Build history of the part. All positions in model axes, mm. Give positions to 0.01 mm unless a question says otherwise; leave off trailing zeros. Loops run counter-clockwise (first coordinate to the right, second up) from the corner with the lowest first, then second, coordinate; pieces in that order, holes last. Notation, with made-up numbers: M 0,86 L 53,86 A18 cw 53,115 Z; hole C 22,-23 d1. An arc over 180 degrees is marked long. Answer as a JSON object with one key per item and string values. Group by question number.
1. Drill centre lines: line 1 along Y through (x, z) = (8, 6.5); line 2 along X through (y, z) = (-54, -9.75); line 3 along X through (y, z) = (51, -2). Where is each one in solid material? Low to high. Write a range as [from, to].
2. Slice it at A-A (x = -54.5). List the corners of the cut face in (y, z), then the cut area to 3 significant figures.
3. Slice it at B-B (y = -20). List the corners of the cut face in (x, z), then the cut area to 3 significant figures.
4. Mould opens along Y. For faces 1 (the face through (-6, 54.193, 0)), 2 (the face through (31, 7.468, 0)) say: released by +Y, released by -Y, zero draft, split by the parting line, or undercut.
5. Slice it at D-D (x = -26). List the corners of the cut face in (y, z), then the cut area to 3 significant figures.
6. Slice it at C-C (z = -4.25). Give the number of separate pieces and of enclosed holes in the cut face, then the cut area to 3 significant figures.
7. Drop flat-ended pins along their axis: pin 1 Ø2 at (x, z) = (-5, 5) entering from -Y; pin 2 Ø2 at (x, z) = (6, -1.5) entering from -Y; pin 3 Ø5 at (y, z) = (19.5, 6) entering from +X. Give the stop position or say it passes through.
from build123d import *

# Parameters (mm, degrees)
F0_W     = 34.350958
F0_H     = 4.69392
F0_W_2   = 4.2672
F0_H_2   = 36.697921
F0_W_3   = 32.217363
F0_W_4   = 4.480557
F0_H_3   = 37.12464
F0_H_4   = 34.350963
F0_H_5   = 4.05384
F1_DEPTH = 11.176


with BuildPart() as f1:
    # F0 (on Top) → F1 (new body, symmetric)
    with BuildSketch(Plane.XY):
        with BuildLine():
            ThreePointArc((-12.7, 0), (-8.980256, 8.980256), (0, 12.7))
            Line((0, 12.7), (0, 76.2))
            ThreePointArc((0, 76.2), (-53.881537, 53.881537), (-76.2, 0))
            Line((-76.2, 0), (-12.7, 0))
        make_face()
        with BuildLine():
            Line((-49.08218, 40.288828), (-17.906999, 12.7))
            Line((-17.906999, 12.7), (-62.217039, 12.7))
            ThreePointArc((-62.217039, 12.7), (-57.333802, 27.296247), (-49.08218, 40.288828))
        make_face(mode=Mode.SUBTRACT)
        with Locations((-33.588959, 5.12064)):
            Rectangle(F0_W, F0_H, mode=Mode.SUBTRACT)
        with Locations((-5.958838, 35.844481)):
            Rectangle(F0_W_2, F0_H_2, mode=Mode.SUBTRACT)
        with BuildLine():
            ThreePointArc((-44.31846, 45.476633), (-29.712564, 56.119636), (-12.7, 62.217039))
            Line((-12.7, 62.217039), (-12.7, 17.49552))
            Line((-12.7, 17.49552), (-44.31846, 45.476633))
        make_face(mode=Mode.SUBTRACT)
        with BuildLine():
            ThreePointArc((0, 12.7), (8.980256, 8.980256), (12.7, 0))
            Line((12.7, 0), (76.2, 0))
            ThreePointArc((76.2, 0), (53.881537, 53.881537), (0, 76.2))
            Line((0, 76.2), (0, 12.7))
        make_face()
        with Locations((31.485843, 5.12064)):
            Rectangle(F0_W_3, F0_H, mode=Mode.SUBTRACT)
        with Locations((6.096001, 35.631121)):
            Rectangle(F0_W_4, F0_H_3, mode=Mode.SUBTRACT)
        with BuildLine():
            Line((62.217039, 12.7), (17.724123, 12.7))
            Line((17.724123, 12.7), (42.179105, 47.467601))
            ThreePointArc((42.179105, 47.467601), (55.016682, 31.708276), (62.217039, 12.7))
        make_face(mode=Mode.SUBTRACT)
        with BuildLine():
            Line((36.695692, 51.82351), (12.7, 17.708881))
            Line((12.7, 17.708881), (12.7, 62.217039))
            ThreePointArc((12.7, 62.217039), (25.23866, 58.26886), (36.695692, 51.82351))
        make_face(mode=Mode.SUBTRACT)
        with BuildLine():
            Line((76.2, 0), (12.7, 0))
            ThreePointArc((12.7, 0), (8.980256, -8.980256), (0, -12.7))
            Line((0, -12.7), (0, -76.2))
            ThreePointArc((0, -76.2), (53.881537, -53.881537), (76.2, 0))
        make_face()
        with BuildLine():
            Line((12.7, -62.217039), (12.7, -17.068801))
            Line((12.7, -17.068801), (39.648922, -49.600534))
            ThreePointArc((39.648922, -49.600534), (26.923901, -57.509595), (12.7, -62.217039))
        make_face(mode=Mode.SUBTRACT)
        with Locations((6.096001, -33.390842)):
            Rectangle(F0_W_4, F0_H_4, mode=Mode.SUBTRACT)
        with Locations((31.485843, -4.58724)):
            Rectangle(F0_W_3, F0_H_5, mode=Mode.SUBTRACT)
        with BuildLine():
            Line((45.322148, -44.476431), (17.510762, -12.7))
            Line((17.510762, -12.7), (62.217039, -12.7))
            ThreePointArc((62.217039, -12.7), (56.067857, -29.810156), (45.322148, -44.476431))
        make_face(mode=Mode.SUBTRACT)
        with BuildLine():
            Line((0, -76.2), (0, -12.7))
            ThreePointArc((0, -12.7), (-8.980256, -8.980256), (-12.7, 0))
            Line((-12.7, 0), (-76.2, 0))
            ThreePointArc((-76.2, 0), (-53.881537, -53.881537), (0, -76.2))
        make_face()
        with BuildLine():
            Line((-41.441198, -48.11317), (-12.7, -17.068801))
            Line((-12.7, -17.068801), (-12.7, -62.217039))
            ThreePointArc((-12.7, -62.217039), (-27.974043, -57.006165), (-41.441198, -48.11317))
        make_face(mode=Mode.SUBTRACT)
        with BuildLine():
            Line((-62.217039, -12.7), (-17.48028, -12.7))
            Line((-17.48028, -12.7), (-46.881881, -42.829186))
            ThreePointArc((-46.881881, -42.829186), (-56.591392, -28.803896), (-62.217039, -12.7))
        make_face(mode=Mode.SUBTRACT)
        with Locations((-5.958838, -33.390842)):
            Rectangle(F0_W_2, F0_H_4, mode=Mode.SUBTRACT)
        with Locations((-33.588959, -4.58724)):
            Rectangle(F0_W, F0_H_5, mode=Mode.SUBTRACT)
    extrude(amount=F1_DEPTH, both=True)


solid = f1.part
Established:
{
 "1": {"line 1": "y = [-75.78, -50.57], [-16.22, -9.86], [9.86, 17.07], [54.19, 75.78]", "line 2": "x = [-53.76, -33.41], [-12.7, 12.7], [33.41, 53.76]", "line 3": "x = [-56.62, -37.83], [-12.7, -8.09], [-3.83, 3.86], [8.34, 12.7], [36.12, 56.62]"},
 "2": {"outline": "M -53.26,-11.18 L -32.59,-11.18 L -32.59,11.18 L -53.26,11.18 Z; M -12.7,-11.18 L 12.7,-11.18 L 12.7,11.18 L -12.7,11.18 Z; M 32.59,-11.18 L 53.26,-11.18 L 53.26,11.18 L 32.59,11.18 Z", "area": "1,490 mm^2"},
 "3": {"outline": "M -73.53,-11.18 L -60.27,-11.18 L -60.27,11.18 L -73.53,11.18 Z; M -24.6,-11.18 L -15.41,-11.18 L -15.41,11.18 L -24.6,11.18 Z; M -12.7,-11.18 L -8.09,-11.18 L -8.09,11.18 L -12.7,11.18 Z; M -3.83,-11.18 L 3.86,-11.18 L 3.86,11.18 L -3.83,11.18 Z; M 8.34,-11.18 L 12.7,-11.18 L 12.7,11.18 L 8.34,11.18 Z; M 15.13,-11.18 L 23.9,-11.18 L 23.9,11.18 L 15.13,11.18 Z; M 60.27,-11.18 L 73.53,-11.18 L 73.53,11.18 L 60.27,11.18 Z", "area": "1,370 mm^2"},
 "4": {"face 1": "undercut", "face 2": "undercut"},
 "5": {"outline": "M -71.63,-11.18 L -57.93,-11.18 L -57.93,11.18 L -71.63,11.18 Z; M -31.43,-11.18 L -21.43,-11.18 L -21.43,11.18 L -31.43,11.18 Z; M -12.7,-11.18 L -6.61,-11.18 L -6.61,11.18 L -12.7,11.18 Z; M -2.56,-11.18 L 2.77,-11.18 L 2.77,11.18 L -2.56,11.18 Z; M 7.47,-11.18 L 12.7,-11.18 L 12.7,11.18 L 7.47,11.18 Z; M 19.86,-11.18 L 29.27,-11.18 L 29.27,11.18 L 19.86,11.18 Z; M 57.93,-11.18 L 71.63,-11.18 L 71.63,11.18 L 57.93,11.18 Z", "area": "1,420 mm^2"},
 "6": {"separate pieces": "1", "enclosed holes": "17", "area": "10,900 mm^2"},
 "7": {"pin 1": "stops at y = -76.09", "pin 2": "stops at y = -76.04", "pin 3": "stops at x = 74.28"}
}
